from build123d import *

# Parameters (mm, degrees)
SKETCH4_R           = 37.5
BOSS_EXTRUDE2_DEPTH = 5
SKETCH5_R           = 10
CUT_EXTRUDE1_DEPTH  = 54.268189382
BOSS_EXTRUDE3_DEPTH = 4.75
SKETCH1_R           = 37.5
SKETCH1_R_2         = 26.5
CUT_EXTRUDE2_DEPTH  = 60.397495738


with BuildPart() as part:
    # Sketch4 → Boss-Extrude2 (new body)
    with BuildSketch(Plane.XY):
        Circle(SKETCH4_R)
    extrude(amount=BOSS_EXTRUDE2_DEPTH)

    # Sketch5 → Cut-Extrude1 (cut, through all)
    with BuildSketch(Plane.XY.offset(5)):
        Circle(SKETCH5_R)
    extrude(amount=-CUT_EXTRUDE1_DEPTH, mode=Mode.SUBTRACT)

    # Sketch6 → Boss-Extrude3 (add, symmetric)
    with BuildSketch(Plane(origin=(0, 0, 0), x_dir=(1, 0, 0), z_dir=(0, 1, 0))):
        with BuildLine():
            Line((20.25, 2.896446609), (17.353553391, 0))
            Line((17.353553391, 0), (26.5, 0))
            add(Edge.make_bspline(
                [(25, 26.75), (25, 22.72818992), (24.990050178, 20.542467854), (25.01194908, 14.942357728), (24.774871471, 4.983935506), (26.5, 0)],
                knots=[0, 0, 0, 0, 0.44660472, 0.54660472, 1, 1, 1, 1], degree=3))
            Line((25, 26.75), (20.103553391, 26.75))
            Line((20.103553391, 26.75), (18.75, 25.396446609))
            Line((18.75, 25.396446609), (18.75, 21.103553391))
            Line((18.75, 21.103553391), (20.25, 19.603553391))
            Line((20.25, 19.603553391), (20.25, 2.896446609))
        make_face()
        with BuildLine():
            add(Edge.make_bspline(
                [(25, 26.75), (25, 22.72818992), (24.990050178, 20.542467854), (25.01194908, 14.942357728), (24.774871471, 4.983935506), (26.5, 0)],
                knots=[0, 0, 0, 0, 0.44660472, 0.54660472, 1, 1, 1, 1], degree=3))
            Line((26.5, 0), (26.5, 26.75))
            Line((26.5, 26.75), (25, 26.75))
        make_face()
    boss_extrude3 = extrude(amount=BOSS_EXTRUDE3_DEPTH, both=True)

    # Sketch1 → Cut-Extrude2 (cut, through all)
    with BuildSketch(Plane.XY):
        Circle(SKETCH1_R)
        Circle(SKETCH1_R_2, mode=Mode.SUBTRACT)
    cut_extrude2 = extrude(amount=-CUT_EXTRUDE2_DEPTH, mode=Mode.SUBTRACT)

    # Sketch6_4 → Cut-Revolve1 (revolve, cut)
    with BuildSketch(Plane(origin=(0, 0, 0), x_dir=(1, 0, 0), z_dir=(0, 1, 0))):
        with BuildLine():
            add(Edge.make_bspline(
                [(25, 26.75), (25, 22.72818992), (24.990050178, 20.542467854), (25.01194908, 14.942357728), (24.774871471, 4.983935506), (26.5, 0)],
                knots=[0, 0, 0, 0, 0.44660472, 0.54660472, 1, 1, 1, 1], degree=3))
            Line((26.5, 0), (26.5, 26.75))
            Line((26.5, 26.75), (25, 26.75))
        make_face()
    cut_revolve1 = revolve(axis=Axis((0, 0, 0), (0, 0, -1)), mode=Mode.SUBTRACT)

    # Mirror1: Boss-Extrude3, Cut-Extrude2, Cut-Revolve1 across plane
    add(boss_extrude3.mirror(Plane(origin=(0, 0, 0), x_dir=(0, 0, 1), z_dir=(1, 0, 0))))
    add(cut_extrude2.mirror(Plane(origin=(0, 0, 0), x_dir=(0, 0, 1), z_dir=(1, 0, 0))), mode=Mode.SUBTRACT)
    add(cut_revolve1.mirror(Plane(origin=(0, 0, 0), x_dir=(0, 0, 1), z_dir=(1, 0, 0))), mode=Mode.SUBTRACT)


solid = part.part
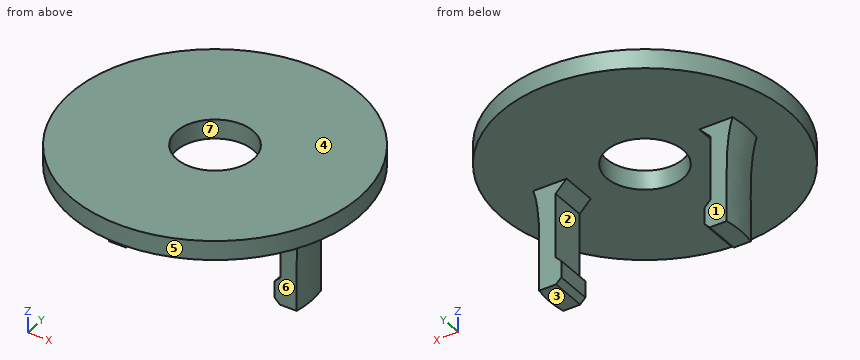
The model under review builds one solid part; all positions refer to its coordinate system, in mm. Face numbers are marked on the shaded views. A direction names the side the tool comes from. Give positions to 0.01 mm unless a question says otherwise; leave off trailing zeros. Write each loop counter-clockwise with the first axis right and the second up, starting at its lowest first coordinate (ties: lowest second). Pieces come first, ordered by that corner, then holes. Notation, with made-up numbers: M -37,30.25 L -23,30.25 A19 cw -23,64.25 Z; hole C -23.75,89.25 d11. An arc over 180 degrees is marked long. One line per question, with ' | ' between items. Start each with the question number.
Item 1: For pin 1 (2.5 mm diameter, centred on x = -21, z = -8.5, fed in from -Y); pin 2 (10.5 mm diameter, centred on y = 2, z = -12.5, fed in from +X); pin 3 (3.5 mm diameter, centred on y = 2, z = -24, fed in from -X); pin 4 (12 mm diameter, centred on x = 0, y = 0, fed in from -Z), all flat-tipped, find the tip position at first contact; note any pin that passes through.
Item 2: We need section D-D on y = -32.5. Write out the cut boundary in (x, z).
Item 3: For the marked faces 1, 2 and 3, list the 3-axis set-ups (+Z, -Z, +X, -X, +Y, -Y) from which the entire face can be reached by the end or side of a thin tool; tool diameter is ignored.
Item 4: We need section C-C on z = 1.5. Write out the cut boundary in (x, y), plus the area to 3 significant figures.
Item 5: We need section B-B on y = 7. Write out the cut boundary in (x, z).
Item 6: Wall thickness on line 1 (Y direction, x = 0, z = 3.15); line 2 (Z direction, x = 4, y = 32); line 3 (Z direction, x = 19, y = -1): over which ranges is each line inside the solid? List them lowest first. Write a range as from..to.
Item 7: Draft analysis for pull direction Y (two halves, no side actions). For the marked faces 4, 5, 6 and 7, state which applies: released by +Y, released by -Y, zero draft, split by the parting line, or undercut.
Item 8: We need section A-A on x = 0. Write out the cut boundary in (y, z).
Results found:
1) pin 1: stops at y = -4.75 | pin 2: stops at x = 25.18 | pin 3: stops at x = -25 | pin 4: passes through
2) outline: M -18.71,0 L 18.71,0 L 18.71,5 L -18.71,5 Z
3) face 1: -Z, +X, -X, +Y | face 2: +Y, -Y | face 3: -Z, +X, -X, +Y, -Y
4) outline: C 0,0 d75; hole C 0,0 d20 | area: 4,100 mm2
5) outline: M -36.84,0 L -7.14,0 L -7.14,5 L -36.84,5 Z; M 7.14,0 L 36.84,0 L 36.84,5 L 7.14,5 Z
6) line 1: y = -37.5..-10, 10..37.5 | line 2: z = 0..5 | line 3: z = -25.65..-20.85, -1.65..5
7) face 4: zero draft | face 5: split by the parting line | face 6: released by -Y | face 7: undercut
8) outline: M -37.5,0 L -10,0 L -10,5 L -37.5,5 Z; M 10,0 L 37.5,0 L 37.5,5 L 10,5 Z
